The listing builds one solid part. Answer for the finished solid, in the listing's coordinates (mm). Face numbers are marked on the shaded views. A direction names the side the tool comes from. Give positions to 0.01 mm unless a question says otherwise; leave off trailing zeros. Write each loop counter-clockwise with the first axis right and the second up, starting at its lowest first coordinate (ties: lowest second). Pieces come first, ordered by that corner, then holes. Notation, with made-up numbers: (-13.5, 22.5) -> (25.5, 22.5) arc R37 ccw to (25.5, 58.5) -> close; hole circle Ø11 at (19, -2). An arc over 180 degrees is marked (long way). Put each result on its own line as item: value. Start each with the question number.
1) A cutting plane is placed at D-D (z = 53.5). Write down the section's boundary in (x, y), then the cut area to 3 significant figures.
2) A cutting plane is placed at B-B (x = -2.5). Write down the section's boundary in (y, z), then the cut area to 3 significant figures.
3) A cutting plane is placed at A-A (z = 39). Write down the section's boundary in (x, y), then the cut area to 3 significant figures.
4) For the marked faces 1, 2, 3 and 4, determine the directions among +Z, -Z, +X, -X, +Y, -Y from which every point of the face is accessible in a straight line to the end or side of a thin tool.
5) A cutting plane is placed at C-C (z = 83.5). Write down the section's boundary in (x, y).
6) Flat-ended cylindrical pins translate along their axes: pin 1 Ø8 at (x, z) = (18.5, 68) entering from -Y; pin 2 Ø3.5 at (x, z) = (55.5, 57.5) entering from +Y; pin 3 Ø3 at (x, z) = (-44, 58) entering from -Y; pin 4 Ø2.5 at (x, z) = (55, 83.5) entering from +Y. Find the tip coordinate at first contact, or state that the pin passes through.
7) Find the intervals of material crossed by line 1 along Z through (x, y) = (55, -5); line 2 along X through (y, z) = (-0.75, 7); line 3 along Y through (x, z) = (-32, 18.5), in increasing order. Write a range as from..to.
from build123d import *

# Parameters (mm, degrees)
EXTRUDE_1_DEPTH     = 90
SKETCH_2_W          = 3
SKETCH_2_H          = 11
SKETCH_2_W_2        = 60
SKETCH_2_H_2        = 40
CUT_EXTRUDE_1_DEPTH = 109.461974904
CUT_EXTRUDE_2_REACH = 110.462
SKETCH_3_R          = 2
FILLET_1_R          = 5
FILLET_2_DEPTH      = 90
FILLET_2_2_DEPTH    = 90
CUT_EXTRUDE_3_REACH = 110.333


with BuildPart() as part:
    # 草图1 → 凸台-拉伸1 (new body)
    with BuildSketch(Plane.XY):
        Polygon((-43, 0), (43, 0), (43, -6), (60, -6), (60, -4), (45, -4), (45, 2), (-45, 2), (-45, -4), (-60, -4), (-60, -6), (-43, -6), align=None)
    extrude(amount=EXTRUDE_1_DEPTH)

    # 草图2 → 切除-拉伸1 (cut, through all)
    with BuildSketch(Plane(origin=(0, 2, 0), x_dir=(1, 0, 0), z_dir=(0, 1, 0))):
        with Locations((51.5, -21)):
            Rectangle(SKETCH_2_W, SKETCH_2_H)
        with Locations((51.5, -68)):
            Rectangle(SKETCH_2_W, SKETCH_2_H)
        with Locations((-51.5, -21)):
            Rectangle(SKETCH_2_W, SKETCH_2_H)
        with Locations((-51.5, -68)):
            Rectangle(SKETCH_2_W, SKETCH_2_H)
        with Locations((-1, -26)):
            Rectangle(SKETCH_2_W_2, SKETCH_2_H_2)
    extrude(amount=-CUT_EXTRUDE_1_DEPTH, mode=Mode.SUBTRACT)

    # 草图3 → 切除-拉伸2 (cut, up to next)
    with BuildSketch(Plane.XZ.offset(6), mode=Mode.PRIVATE) as cut_extrude_2_sk1:
        with Locations((55, 7.5)):
            Circle(SKETCH_3_R)
    cut_extrude_2_tool1 = extrude(cut_extrude_2_sk1.sketch, amount=-CUT_EXTRUDE_2_REACH, mode=Mode.PRIVATE) & part.part
    # 草图3 → 切除-拉伸2 (cut, up to next)
    with BuildSketch(Plane.XZ.offset(6), mode=Mode.PRIVATE) as cut_extrude_2_sk2:
        with Locations((55, 83.5)):
            Circle(SKETCH_3_R)
    cut_extrude_2_tool2 = extrude(cut_extrude_2_sk2.sketch, amount=-CUT_EXTRUDE_2_REACH, mode=Mode.PRIVATE) & part.part
    # 草图3 → 切除-拉伸2 (cut, up to next)
    with BuildSketch(Plane.XZ.offset(6), mode=Mode.PRIVATE) as cut_extrude_2_sk3:
        with Locations((-55, 83.5)):
            Circle(SKETCH_3_R)
    cut_extrude_2_tool3 = extrude(cut_extrude_2_sk3.sketch, amount=-CUT_EXTRUDE_2_REACH, mode=Mode.PRIVATE) & part.part
    # 草图3 → 切除-拉伸2 (cut, up to next)
    with BuildSketch(Plane.XZ.offset(6), mode=Mode.PRIVATE) as cut_extrude_2_sk4:
        with Locations((-55, 7.5)):
            Circle(SKETCH_3_R)
    cut_extrude_2_tool4 = extrude(cut_extrude_2_sk4.sketch, amount=-CUT_EXTRUDE_2_REACH, mode=Mode.PRIVATE) & part.part
    add(cut_extrude_2_tool1.solids().sort_by_distance((55, -6, 7.5))[0], mode=Mode.SUBTRACT)
    add(cut_extrude_2_tool2.solids().sort_by_distance((55, -6, 83.5))[0], mode=Mode.SUBTRACT)
    add(cut_extrude_2_tool3.solids().sort_by_distance((-55, -6, 83.5))[0], mode=Mode.SUBTRACT)
    add(cut_extrude_2_tool4.solids().sort_by_distance((-55, -6, 7.5))[0], mode=Mode.SUBTRACT)

    # 圆角1
    fillet_1_edges = [part.edges().sort_by_distance(p)[0] for p in [
        (60, -5, 0),
        (-60, -5, 0),
        (60, -5, 90),
        (-60, -5, 90),
    ]]
    fillet(fillet_1_edges, radius=FILLET_1_R)

    # 圆角2: read off the stored shape, not the designer's step
    # 圆角2 outline → 圆角2 (cut)
    with BuildSketch(Plane.XY):
        with BuildLine():
            Line((-43, -6), (-43, -3))
            ThreePointArc((-43, -3), (-43.878679656, -5.121320344), (-46, -6))
            Line((-46, -6), (-43, -6))
        make_face()
        with BuildLine():
            ThreePointArc((46, -6), (43.878679656, -5.121320344), (43, -3))
            Line((43, -3), (43, -6))
            Line((43, -6), (46, -6))
        make_face()
        with BuildLine():
            Line((45, 2), (42, 2))
            ThreePointArc((42, 2), (44.121320344, 1.121320344), (45, -1))
            Line((45, -1), (45, 2))
        make_face()
        with BuildLine():
            ThreePointArc((-45, -1), (-44.121320344, 1.121320344), (-42, 2))
            Line((-42, 2), (-45, 2))
            Line((-45, 2), (-45, -1))
        make_face()
    extrude(amount=FILLET_2_DEPTH, mode=Mode.SUBTRACT)

    # Fillet 2 2 outline → Fillet 2 2 (add)
    with BuildSketch(Plane.XY):
        with BuildLine():
            ThreePointArc((-43, -3), (-42.121320344, -0.878679656), (-40, 0))
            Line((-40, 0), (-43, 0))
            Line((-43, 0), (-43, -3))
        make_face()
        with BuildLine():
            ThreePointArc((40, 0), (42.121320344, -0.878679656), (43, -3))
            Line((43, -3), (43, 0))
            Line((43, 0), (40, 0))
        make_face()
        with BuildLine():
            Line((-45, -4), (-45, -1))
            ThreePointArc((-45, -1), (-45.878679656, -3.121320344), (-48, -4))
            Line((-48, -4), (-45, -4))
        make_face()
        with BuildLine():
            ThreePointArc((48, -4), (45.878679656, -3.121320344), (45, -1))
            Line((45, -1), (45, -4))
            Line((45, -4), (48, -4))
        make_face()
    extrude(amount=FILLET_2_2_DEPTH)

    # 草图4 → 切除-拉伸3 (cut, up to next)
    with BuildSketch(Plane(origin=(0, -4, 0), x_dir=(1, 0, 0), z_dir=(0, 1, 0)), mode=Mode.PRIVATE) as cut_extrude_3_sk1:
        Polygon((60, -27), (57, -34), (57, -56), (60, -63), align=None)
    cut_extrude_3_tool1 = extrude(cut_extrude_3_sk1.sketch, amount=-CUT_EXTRUDE_3_REACH, mode=Mode.PRIVATE) & part.part
    # 草图4 → 切除-拉伸3 (cut, up to next)
    with BuildSketch(Plane(origin=(0, -4, 0), x_dir=(1, 0, 0), z_dir=(0, 1, 0)), mode=Mode.PRIVATE) as cut_extrude_3_sk2:
        Polygon((-60, -63), (-57, -56), (-57, -34), (-60, -27), align=None)
    cut_extrude_3_tool2 = extrude(cut_extrude_3_sk2.sketch, amount=-CUT_EXTRUDE_3_REACH, mode=Mode.PRIVATE) & part.part
    add(cut_extrude_3_tool1.solids().sort_by_distance((58.62069, -4, 45))[0], mode=Mode.SUBTRACT)
    add(cut_extrude_3_tool2.solids().sort_by_distance((-58.62069, -4, 45))[0], mode=Mode.SUBTRACT)


solid = part.part
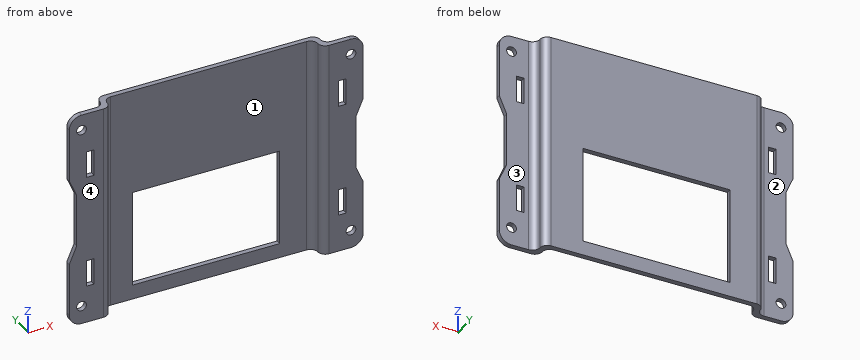
Reply:
1. outline: (-57, -6) -> (-46, -6) arc R3 ccw to (-43, -3) arc R3 cw to (-40, 0) -> (40, 0) arc R3 cw to (43, -3) arc R3 ccw to (46, -6) -> (57, -6) -> (57, -4) -> (48, -4) arc R3 cw to (45, -1) arc R3 ccw to (42, 2) -> (-42, 2) arc R3 ccw to (-45, -1) arc R3 cw to (-48, -4) -> (-57, -4) -> close
1. area: 252 mm2
2. outline: (0, 0) -> (2, 0) -> (2, 6) -> (0, 6) -> close; (0, 46) -> (2, 46) -> (2, 90) -> (0, 90) -> close
2. area: 100 mm2
3. outline: (-57, -6) -> (-46, -6) arc R3 ccw to (-43, -3) arc R3 cw to (-40, 0) -> (-31, 0) -> (-31, 2) -> (-42, 2) arc R3 ccw to (-45, -1) arc R3 cw to (-48, -4) -> (-57, -4) -> close; (29, 0) -> (40, 0) arc R3 cw to (43, -3) arc R3 ccw to (46, -6) -> (57, -6) -> (57, -4) -> (48, -4) arc R3 cw to (45, -1) arc R3 ccw to (42, 2) -> (29, 2) -> close
3. area: 132 mm2
4. face 1: +Z, -Z, -Y
4. face 2: +Z, -Z, -X, +Y
4. face 3: +Z, -Z, +X, +Y
4. face 4: +Z, -Z, +X, -X, -Y
5. outline: (-60, -6) -> (-57, -6) -> (-57, -4) -> (-60, -4) -> close; (-53, -6) -> (-46, -6) arc R3 ccw to (-43, -3) arc R3 cw to (-40, 0) -> (40, 0) arc R3 cw to (43, -3) arc R3 ccw to (46, -6) -> (53, -6) -> (53, -4) -> (48, -4) arc R3 cw to (45, -1) arc R3 ccw to (42, 2) -> (-42, 2) arc R3 ccw to (-45, -1) arc R3 cw to (-48, -4) -> (-53, -4) -> close; (57, -6) -> (60, -6) -> (60, -4) -> (57, -4) -> close
6. pin 1: stops at y = 0
6. pin 2: stops at y = -4
6. pin 3: stops at y = -5.96
6. pin 4: passes through
7. line 1: z = 0..5.5, 9.5..81.5, 85.5..90
7. line 2: x = -44.99..-41.98, 41.98..44.99
7. line 3: y = 0..2
